Autodesk Inventor part; units mm, degrees
ref_plane "YZ Plane" through (0, 0, 0) normal (1, 0, 0) x (0, 1, 0)
ref_plane "XZ Plane" through (0, 0, 0) normal (0, 1, 0) x (-1, 0, 0)
ref_plane "XY Plane" through (0, 0, 0) normal (0, 0, 1) x (1, 0, 0)
sketch "Sketch10" plane through (0, 0, 0) normal (0, 0, 1) x (1, 0, 0)
  circle A0 centre (0, 0) radius 14.3
  dimension "d33" = 28.6
extrude "Extrusion6" add sketch "Sketch10" along normal blind 17.6
sketch "Sketch11" plane through (0, 0, 17.6) normal (0, 0, 1) x (1, 0, 0)
  circle A0 centre (0, 0) radius 12.5
  circle A1 centre (0, 0) radius 14.3
  dimension "d36" = 1.8
extrude "Extrusion7" cut sketch "Sketch11" against normal blind 17 contours A0
sketch "Sketch12" plane through (0, 0, 17.6) normal (0, 0, 1) x (1, 0, 0)
  circle A0 centre (0, 0) radius 12.5
  line L0 (2.5, 7.5) -> (-2.5, 7.5)
  line L1 (-2.5, 7.5) -> (-2.5, 12.5)
  line L2 (-2.5, 12.5) -> (2.5, 12.5)
  line L3 (2.5, 12.5) -> (2.5, 7.5)
  line L4 (2.5, -7.5) -> (-2.5, -7.5)
  line L5 (-2.5, -7.5) -> (-2.5, -12.5)
  line L6 (-2.5, -12.5) -> (2.5, -12.5)
  line L7 (2.5, -12.5) -> (2.5, -7.5)
  dimension "d41" = 5
  dimension "d42" = 5
  dimension "d43" = 5
  dimension "d46" = 5
  dimension "d47" = 5
  dimension "d48" = 5
extrude "Extrusion8" add sketch "Sketch12" against normal blind 8 contours L3 L0 L1 A0 | A0 L2 L3 | L7 L6 A0 | A0 L5 L4 L7 | A0 L1 L2 | L6 L5 A0
sketch "Sketch18" plane through (2.5, 7.5, 17.6) normal (1, 0, 0) x (0, 0, -1)
  line L0 (0, 4.7474) -> (0, 0)
  line L1 (0, 0) -> (3, 0)
  line L2 (0, 0) -> (8, 0)
  line L3 (8, 5) -> (8, 4.7474)
  line L4 (3, 0) -> (8, 4.7474)
  line L5 (8, 4.7474) -> (8, 0)
  line L6 (8, 0) -> (3, 0)
  line L7 (0, -15) -> (8, -15)
  line L8 (0, -15) -> (3, -15)
  line L9 (0, -19.7474) -> (8, -19.7474)
  line L10 (3, -15) -> (8, -19.7474)
  line L11 (8, -19.7474) -> (8, -15)
  line L12 (8, -15) -> (3, -15)
  point P0 (17.6, -7.5)
  dimension "d56" = 3
  dimension "d57" = 3
extrude "Extrusion9" cut sketch "Sketch18" against normal blind 5
sketch "Sketch19" plane through (0, 0, 17.6) normal (0, 0, 1) x (1, 0, 0)
  line L0 (2.5, 7.5) -> (-2.5, 7.5)
  arc A0 (2.5, 12.2474) -> (-2.5, 12.2474) centre (0, 0) ccw
  line L1 (-2.5, 7.5) -> (-2.5, 12.2474)
  line L2 (2.5, -7.5) -> (-2.5, -7.5)
  line L3 (-2.5, -7.5) -> (-2.5, -12.2474)
  point P0 (0, 10)
  point P1 (0, -10)
  dimension "d60" = 2.5
  dimension "d61" = 2.5
  dimension "d63" = 2.5
  dimension "d64" = 2.5
hole "Hole2" at (0, 10, 17.6) at (0, -10, 17.6) direction (0, 0, -1) diameter 2.4 depth 10 tip angle 118
chamfer "Chamfer2" distance 0.6 angle 45 2 edges at (0, -8.8, 17.6) (0, 11.2, 17.6)
properties part number "Clock Dot"
Geometry: final body of the model. Coordinates: model frame, mm. A direction names the side the tool comes from. Round coordinates to 2 decimals unless told otherwise and drop trailing zeros. Loops run counter-clockwise (first coordinate to the right, second up) from the corner with the lowest first, then second, coordinate; pieces in that order, holes last. Notation, with made-up numbers: (-38.5, 2) -> (-4.5, 2) arc R19 cw to (-4.5, 23) -> close; hole circle Ø3 at (2.25, 16.5). An arc over 180 degrees is marked (long way). Use one line per item in the form item = value.
Item 1: Cut plane C-C on y = 0. Output: boundary loops of the cut face in (x, z), then the cut area to 3 significant figures.
Evaluation:
outline = (-14.3, 0) -> (14.3, 0) -> (14.3, 17.6) -> (12.5, 17.6) -> (12.5, 0.6) -> (-12.5, 0.6) -> (-12.5, 17.6) -> (-14.3, 17.6) -> close
area = 78.4 mm2
Item 2: Contact query for flat-ended pins moving along their axis: pin 1 Ø10 at (x, y) = (8.5, -0.5) entering from +Z; pin 2 Ø2.5 at (y, z) = (-9.5, 13.5) entering from -X; pin 3 Ø3 at (x, y) = (0, -10) entering from +Z; pin 4 Ø1.5 at (x, z) = (-2.5, 11.5) entering from +Y. Output: stop coordinate, or through.
Evaluation:
pin_1 = 17.6
pin_2 = -11.68
pin_3 = 17.3
pin_4 = 14.19
Item 3: Cut plane B-B on x = 0. Output: boundary loops of the cut face in (y, z).
Evaluation:
outline = (-14.3, 0) -> (14.3, 0) -> (14.3, 17.6) -> (11.8, 17.6) -> (11.2, 17) -> (11.2, 10.7) -> (12.25, 9.6) -> (12.5, 9.6) -> (12.5, 0.6) -> (-12.5, 0.6) -> (-12.5, 9.6) -> (-12.25, 9.6) -> (-11.2, 10.7) -> (-11.2, 17) -> (-11.8, 17.6) -> (-14.3, 17.6) -> close; (-8.8, 13.23) -> (-7.5, 14.6) -> (-7.5, 17.6) -> (-8.2, 17.6) -> (-8.8, 17) -> close; (7.5, 14.6) -> (8.8, 13.23) -> (8.8, 17) -> (8.2, 17.6) -> (7.5, 17.6) -> close
Item 4: Material intervals for probe 1 along X at (y, z) = (10, 13.25); probe 2 along Y at (x, z) = (0, 14.75); probe 3 along Y at (x, z) = (0, 13.5), sorted ascending.
Evaluation:
probe_1 = -10.22 to -7.5, -2.5 to -1.2, 1.2 to 2.5, 7.5 to 10.22
probe_2 = -14.3 to -11.2, -8.8 to -7.5, 7.5 to 8.8, 11.2 to 14.3
probe_3 = -14.3 to -11.2, -8.8 to -8.54, 8.54 to 8.8, 11.2 to 14.3
Item 5: Access query for faces 5 (the flat face through (2.5, -10, 15)), 6 (the flat face through (0.591, -8.785, 13.246)), 7 (the flat face through (0, 0, 0)). Directions: +Z, -Z, +X, -X, +Y, -Y. A direction counts if a zero-diameter tool reaches every point of the face in a straight line with its end or side. Return the directions, or none.
Evaluation:
face_5 = +Z
face_6 = none
face_7 = -Z, +X, -X, +Y, -Y
Item 6: Cut plane A-A on y = -10. Output: boundary loops of the cut face in (x, z), then the cut area to 3 significant figures.
Evaluation:
outline = (-10.22, 0) -> (10.22, 0) -> (10.22, 17.6) -> (7.5, 17.6) -> (7.5, 0.6) -> (-7.5, 0.6) -> (-7.5, 17.6) -> (-10.22, 17.6) -> close; (-2.5, 11.97) -> (-1.2, 11.97) -> (-1.2, 17) -> (-1.8, 17.6) -> (-2.5, 17.6) -> close; (1.2, 11.97) -> (2.5, 11.97) -> (2.5, 17.6) -> (1.8, 17.6) -> (1.2, 17) -> close
area = 119 mm2
Item 7: Cut plane D-D on x = -6. Output: boundary loops of the cut face in (y, z).
Evaluation:
outline = (-12.98, 0) -> (12.98, 0) -> (12.98, 17.6) -> (10.97, 17.6) -> (10.97, 0.6) -> (-10.97, 0.6) -> (-10.97, 17.6) -> (-12.98, 17.6) -> close
Item 8: Draft query along Y for faces 1 (the cylindrical face through (-1.86, -14.18, 8.68)), 2 (the flat face through (0, 7.5, 16)), 3 (the flat face through (1, -8, 17.6)), 4 (the cylindrical face through (5.77, -11.09, 9.22)). Return one class per face: released by +Y, released by -Y, zero draft, split by the parting line, or undercut.
Evaluation:
face_1 = split by the parting line
face_2 = undercut
face_3 = zero draft
face_4 = undercut
